Part print with two shaded views. Sizes in mm from the minimum x, y, z corner. Round coordinates to 2 decimals unless told otherwise and drop trailing zeros. Write each loop counter-clockwise with the first axis right and the second up, starting at its lowest first coordinate (ties: lowest second). Pieces come first, ordered by that corner, then holes. Notation, with made-up numbers: (65.25, 16.25) - (94.25, 16.25) arc R38 cw to (94.25, 54.25) - close; hole circle Ø11 at (4, 65.5). An arc over 180 degrees is marked (long way). Use one line per item in the form item = value. Start each with the question number.
Item 1: Drill centre lines: L1, parallel to X at y = 50, z = 2.75; L2, parallel to Y at x = 68, z = 2.8; L3, parallel to Y at x = 164, z = 2.6. Where is each one in solid material? Low to high.
Item 2: Band-saw the part on B-B, the plane z = 3. Give the number of separate pieces and of enclosed holes in the cut face, and give its area (3 significant figures).
Item 3: Band-saw the part on A-A, the plane x = 115. List the corners of the cut face in (y, z).
Item 4: Pin check, flat tip, straight feed: pin 1 (2.5 mm diameter, centred on x = 68, y = 50, fed in from +Z). Stop position of the tip, or through.
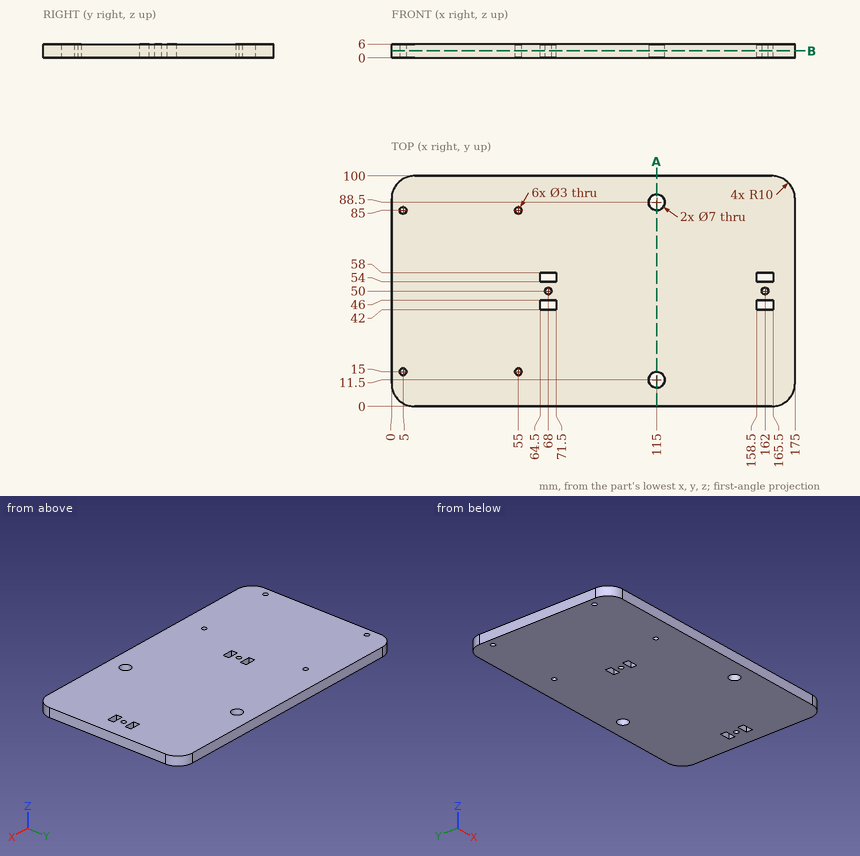
Determined:
q1.L1 = 0 to 66.5, 69.5 to 160.5, 163.5 to 175
q1.L2 = 0 to 42, 46 to 48.5, 51.5 to 54, 58 to 100
q1.L3 = 0 to 42, 46 to 54, 58 to 100
q2.separate_pieces = 1
q2.enclosed_holes = 12
q2.area = 17,200 mm²
q3.outline = (0, 0) - (8, 0) - (8, 6) - (0, 6) - close; (15, 0) - (85, 0) - (85, 6) - (15, 6) - close; (92, 0) - (100, 0) - (100, 6) - (92, 6) - close
q4.pin_1 = through
